Work out the finished part from the listing and answer in its coordinate system (mm). Give positions to 0.01 mm unless a question says otherwise; leave off trailing zeros. Loops run counter-clockwise (first coordinate to the right, second up) from the corner with the lowest first, then second, coordinate; pieces in that order, holes last. Notation, with made-up numbers: (3.25, 84.5) - (62.25, 84.5) arc R4 ccw to (62.25, 91.5) - close; hole circle Ø8 at (-0.75, 35.25). An arc over 180 degrees is marked (long way). One line per question, with ' | ' between items.
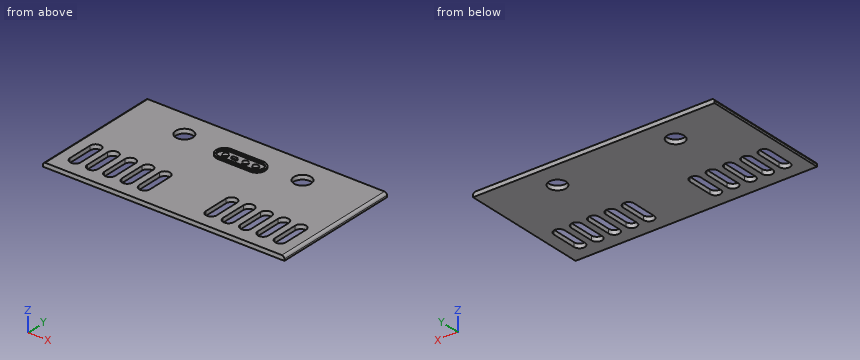
from build123d import *

# Parameters (mm, degrees)
SKETCH1_W           = 280
SKETCH1_H           = 150
BOSS_EXTRUDE1_DEPTH = 5
FILLET1_R           = 3
BOSS_EXTRUDE2_DEPTH = 2
SKETCH4_R           = 3.25
BOSS_EXTRUDE3_DEPTH = 1
CUT_EXTRUDE1_DEPTH  = 5
CUT_EXTRUDE2_REACH  = 160.902
SKETCH6_R           = 10


with BuildPart() as part:
    # Sketch1 → Boss-Extrude1 (new body)
    with BuildSketch(Plane.XY):
        Rectangle(SKETCH1_W, SKETCH1_H)
    extrude(amount=BOSS_EXTRUDE1_DEPTH)

    # Fillet1
    fillet1_edges = [part.edges().sort_by_distance(p)[0] for p in [
        (140, 0, 5),
        (-140, 0, 5),
    ]]
    fillet(fillet1_edges, radius=FILLET1_R)

    # Sketch2 → Boss-Extrude2 (add)
    with BuildSketch(Plane.XY.offset(5)):
        with BuildLine():
            Line((-18.760224692, 47.124562697), (18.760224692, 47.124562697))
            ThreePointArc((18.760224692, 47.124562697), (28.384787389, 37.5), (18.760224692, 27.875437303))
            Line((18.760224692, 27.875437303), (-18.760224692, 27.875437303))
            ThreePointArc((-18.760224692, 27.875437303), (-28.384787389, 37.5), (-18.760224692, 47.124562697))
        make_face()
        with BuildLine():
            Line((-18.760224692, 45.124562697), (18.760224692, 45.124562697))
            ThreePointArc((18.760224692, 45.124562697), (26.384787389, 37.5), (18.760224692, 29.875437303))
            Line((18.760224692, 29.875437303), (-18.760224692, 29.875437303))
            ThreePointArc((-18.760224692, 29.875437303), (-26.384787389, 37.5), (-18.760224692, 45.124562697))
        make_face(mode=Mode.SUBTRACT)
    extrude(amount=BOSS_EXTRUDE2_DEPTH)

    # Sketch4 → Boss-Extrude3 (add)
    with BuildSketch(Plane.XY.offset(5)):
        with Locations((17.470523742, 37.5)):
            Circle(SKETCH4_R)
        with Locations((-17.4898287, 37.5)):
            Circle(SKETCH4_R)
        with Locations((5.652243355, 37.5)):
            Circle(SKETCH4_R)
        with BuildLine():
            Line((-8.935173859, 39.13468348), (-4.880366362, 39.13468348))
            ThreePointArc((-4.880366362, 39.13468348), (-3.245682882, 37.5), (-4.880366362, 35.86531652))
            Line((-4.880366362, 35.86531652), (-8.935173859, 35.86531652))
            ThreePointArc((-8.935173859, 35.86531652), (-10.569857339, 37.5), (-8.935173859, 39.13468348))
        make_face()
    extrude(amount=BOSS_EXTRUDE3_DEPTH)

    # Sketch5 → Cut-Extrude1 (cut)
    with BuildSketch(Plane.XY.offset(5)):
        with BuildLine():
            Line((125.208389031, -24.677314769), (125.208389031, -54.157596843))
            ThreePointArc((125.208389031, -54.157596843), (118.914845667, -60.451140207), (112.621302303, -54.157596843))
            Line((112.621302303, -54.157596843), (112.621302303, -24.677314769))
            ThreePointArc((112.621302303, -24.677314769), (118.914845667, -18.383771405), (125.208389031, -24.677314769))
        make_face()
        with BuildLine():
            Line((105.142389031, -24.677314769), (105.142389031, -54.157596843))
            ThreePointArc((105.142389031, -54.157596843), (98.848845667, -60.451140207), (92.555302303, -54.157596843))
            Line((92.555302303, -54.157596843), (92.555302303, -24.677314769))
            ThreePointArc((92.555302303, -24.677314769), (98.848845667, -18.383771405), (105.142389031, -24.677314769))
        make_face()
        with BuildLine():
            Line((85.076389031, -24.677314769), (85.076389031, -54.157596843))
            ThreePointArc((85.076389031, -54.157596843), (78.782845667, -60.451140207), (72.489302303, -54.157596843))
            Line((72.489302303, -54.157596843), (72.489302303, -24.677314769))
            ThreePointArc((72.489302303, -24.677314769), (78.782845667, -18.383771405), (85.076389031, -24.677314769))
        make_face()
        with BuildLine():
            Line((65.010389031, -24.677314769), (65.010389031, -54.157596843))
            ThreePointArc((65.010389031, -54.157596843), (58.716845667, -60.451140207), (52.423302303, -54.157596843))
            Line((52.423302303, -54.157596843), (52.423302303, -24.677314769))
            ThreePointArc((52.423302303, -24.677314769), (58.716845667, -18.383771405), (65.010389031, -24.677314769))
        make_face()
        with BuildLine():
            Line((44.944389031, -24.677314769), (44.944389031, -54.157596843))
            ThreePointArc((44.944389031, -54.157596843), (38.650845667, -60.451140207), (32.357302303, -54.157596843))
            Line((32.357302303, -54.157596843), (32.357302303, -24.677314769))
            ThreePointArc((32.357302303, -24.677314769), (38.650845667, -18.383771405), (44.944389031, -24.677314769))
        make_face()
    cut_extrude1 = extrude(amount=-CUT_EXTRUDE1_DEPTH, mode=Mode.SUBTRACT)

    # Mirror1: Cut-Extrude1 across plane
    add(cut_extrude1.mirror(Plane(origin=(0, 0, 0), x_dir=(0, 0, 1), z_dir=(1, 0, 0))), mode=Mode.SUBTRACT)

    # Sketch6 → Cut-Extrude2 (cut, up to next)
    with BuildSketch(Plane.XY.offset(5), mode=Mode.PRIVATE) as cut_extrude2_sk1:
        with Locations((65.764998976, 45)):
            Circle(SKETCH6_R)
    cut_extrude2_tool1 = extrude(cut_extrude2_sk1.sketch, amount=-CUT_EXTRUDE2_REACH, mode=Mode.PRIVATE) & part.part
    # Sketch6 → Cut-Extrude2 (cut, up to next)
    with BuildSketch(Plane.XY.offset(5), mode=Mode.PRIVATE) as cut_extrude2_sk2:
        with Locations((-71.235001024, 45)):
            Circle(SKETCH6_R)
    cut_extrude2_tool2 = extrude(cut_extrude2_sk2.sketch, amount=-CUT_EXTRUDE2_REACH, mode=Mode.PRIVATE) & part.part
    add(cut_extrude2_tool1.solids().sort_by_distance((65.764999, 45, 5))[0], mode=Mode.SUBTRACT)
    add(cut_extrude2_tool2.solids().sort_by_distance((-71.235001, 45, 5))[0], mode=Mode.SUBTRACT)


solid = part.part
1. Find section C-C on y = 7.5. Write down the section's boundary in (x, z).
Evaluation:
outline: (-140, 0) - (140, 0) - (140, 2) arc R3 ccw to (137, 5) - (-137, 5) arc R3 ccw to (-140, 2) - close
2. Find section B-B on y = -50. State how many separate pieces and enclosed holes the cut face has, then the cut area to 3 significant figures.
Evaluation:
separate pieces: 11 | enclosed holes: 0 | area: 767 mm2
3. Find section D-D on x = 90. Write down the section's boundary in (y, z), then the cut area to 3 significant figures.
Evaluation:
outline: (-75, 0) - (75, 0) - (75, 5) - (-75, 5) - close | area: 750 mm2
4. Flat-ended cylindrical pins translate along their axes: pin 1 (2 mm diameter, centred on y = 16, z = 3.5, fed in from +X); pin 2 (1 mm diameter, centred on x = 8.5, z = 6, fed in from -Y); pin 3 (12 mm diameter, centred on x = 53, y = -21, fed in from +Z); pin 4 (3 mm diameter, centred on x = 48, z = 6, fed in from +Y). Find the tip coordinate at first contact, or state that the pin passes through.
Evaluation:
pin 1: x = 139.96 | pin 2: y = 27.88 | pin 3: z = 5 | pin 4: y = 75
5. Consider L1, parallel to Y at x = 79, z = 3; L2, parallel to Y at x = -71.5, z = 4.75; L3, parallel to Z at x = 108.5, y = -55.5. Determine where each line is inside the solid, lowest interval first.
Evaluation:
L1: -75 to -60.45, -18.39 to 75 | L2: -75 to 35, 55 to 75 | L3: 0 to 5
6. Find section A-A on x = -100.5. Write down the section's boundary in (y, z).
Evaluation:
outline: (-75, 0) - (-60.23, 0) - (-60.23, 5) - (-75, 5) - close; (-18.6, 0) - (75, 0) - (75, 5) - (-18.6, 5) - close
